The model under review builds one solid part; all positions refer to its coordinate system, in mm. A direction names the side the tool comes from. Coordinates: 2 decimals unless noted, no trailing zeros. Write each loop counter-clockwise with the first axis right and the second up, starting at its lowest first coordinate (ties: lowest second). Pieces come first, ordered by that corner, then holes.
```python
from build123d import *

# Parameters (mm, degrees)
BOSS_EXTRUDE1_START = 19.16
SKETCH1_W           = 90
SKETCH1_H           = 100
SKETCH1_R           = 2.5
SKETCH1_R_2         = 3.57
BOSS_EXTRUDE1_DEPTH = 3.18
FILLET1_R           = 10
SKETCH2_R           = 2.5
CUT_EXTRUDE1_DEPTH  = 10
SKETCH3_W           = 21.4
SKETCH3_H           = 22.810510703
CUT_EXTRUDE2_DEPTH  = 72.134467033


with BuildPart() as part:
    # Sketch1 → Boss-Extrude1 (new body)
    with BuildSketch(Plane.XY.offset(BOSS_EXTRUDE1_START)):
        with Locations((0, -5)):
            Rectangle(SKETCH1_W, SKETCH1_H)
        with Locations((32.3, -42.3)):
            Circle(SKETCH1_R, mode=Mode.SUBTRACT)
        with Locations((-32.3, -42.3)):
            Circle(SKETCH1_R_2, mode=Mode.SUBTRACT)
        with Locations((-32.3, 32.3)):
            Circle(SKETCH1_R_2, mode=Mode.SUBTRACT)
        with Locations((32.3, 32.3)):
            Circle(SKETCH1_R, mode=Mode.SUBTRACT)
    extrude(amount=-BOSS_EXTRUDE1_DEPTH)

    # Fillet1
    fillet1_edges = [part.edges().sort_by_distance(p)[0] for p in [
        (-45, 45, 17.57),
        (45, 45, 17.57),
        (45, -55, 17.57),
        (-45, -55, 17.57),
    ]]
    fillet(fillet1_edges, radius=FILLET1_R)

    # Sketch2 → Cut-Extrude1 (cut)
    with BuildSketch(Plane.XY.offset(19.16)):
        with Locations((10, -5)):
            Circle(SKETCH2_R)
        with Locations((-10, -5)):
            Circle(SKETCH2_R)
    extrude(amount=-CUT_EXTRUDE1_DEPTH, mode=Mode.SUBTRACT)

    # Sketch3 → Cut-Extrude2 (cut, through all)
    with BuildSketch(Plane(origin=(0, 0, 15.98), x_dir=(-1, 0, 0), z_dir=(0, 0, -1))):
        with Locations((-0.5, 16.405255352)):
            Rectangle(SKETCH3_W, SKETCH3_H)
        with Locations((-0.5, -26.405255352)):
            Rectangle(SKETCH3_W, SKETCH3_H)
    extrude(amount=-CUT_EXTRUDE2_DEPTH, mode=Mode.SUBTRACT)


solid = part.part
```
Item 1: Mouldability with a two-part tool opening along Y and no side actions: class faces 1 (the face through (45, -6, 18)), 2 (the face through (0, -55, 18)), 3 (the face through (11.2, 16, 18)) as pulls with the +Y half, pulls with the -Y half, needs draft (parallel to the pull), parting line crosses it, or undercut.
Solved:
face 1: needs draft
face 2: pulls with the -Y half
face 3: undercut
Item 2: Take a section at C-C, the plane z = 18.1. Count the separate pieces of the cut face and the enclosed holes in it, plus the area to 3 significant figures.
Solved:
separate pieces: 1
enclosed holes: 8
area: 7,780 mm2
Item 3: Take a section at A-A, the plane y = 24.5. Write out the cut boundary in (x, z), plus the area to 3 significant figures.
Solved:
outline: (-45, 15.98) - (-10.2, 15.98) - (-10.2, 19.16) - (-45, 19.16) - close; (11.2, 15.98) - (45, 15.98) - (45, 19.16) - (11.2, 19.16) - close
area: 218 mm2
Item 4: To check wall thickness, follow line 1 along Y through (x, z) = (-10, 17.1); line 2 along Y through (x, z) = (32.3, 18.5); line 3 along Y through (x, z) = (4.5, 17.1). State the ranges of each line that lie inside material, in increasing order.
Solved:
line 1: y = -55 to -37.81, -15 to -7.5, -2.5 to 5, 27.81 to 45
line 2: y = -55 to -44.8, -39.8 to 29.8, 34.8 to 45
line 3: y = -55 to -37.81, -15 to 5, 27.81 to 45
Item 5: Take a section at D-D, the plane y = -5. Write out the cut boundary in (x, z).
Solved:
outline: (-45, 15.98) - (-12.5, 15.98) - (-12.5, 19.16) - (-45, 19.16) - close; (-7.5, 15.98) - (7.5, 15.98) - (7.5, 19.16) - (-7.5, 19.16) - close; (12.5, 15.98) - (45, 15.98) - (45, 19.16) - (12.5, 19.16) - close
Item 6: Take a section at B-B, the plane x = 32.3. Write out the cut boundary in (y, z).
Solved:
outline: (-55, 15.98) - (-44.8, 15.98) - (-44.8, 19.16) - (-55, 19.16) - close; (-39.8, 15.98) - (29.8, 15.98) - (29.8, 19.16) - (-39.8, 19.16) - close; (34.8, 15.98) - (45, 15.98) - (45, 19.16) - (34.8, 19.16) - close
Item 7: Machinability: for faces 4 (the face through (-42.15, -51.99, 17.55)), 5 (the face through (1, 27.811, 18)), which of the approach directions +Z, -Z, +X, -X, +Y, -Y give a long, thin tool a straight path to every point of the face, cutting with its end or side? Answer none if there is none.
Solved:
face 4: +Z, -Z, -X, -Y
face 5: +Z, -Z
